from build123d import *

# Parameters (mm, degrees)
PROFILE_SKETCH_R              = 20.6375
PROFILE_EXTRUDE_DEPTH         = 3.175
BORE_SKETCH_R                 = 14.4145
BORE_CUT_DEPTH                = 4.175
BOLT_CLEARANCE_SKETCH_R       = 1.4732
BOLT_CLEARANCE_CUT_DEPTH      = 4.175
BOLT_HEAD_CLEARANCE_SKETCH_R  = 2.4511
BOLT_HEAD_CLEARANCE_CUT_DEPTH = 4.175


with BuildPart() as part:
    # Profile Sketch → Profile Extrude (new body)
    with BuildSketch(Plane(origin=(0, 0, 0), x_dir=(1, 0, 0), z_dir=(0, 1, 0))):
        Circle(PROFILE_SKETCH_R)
    extrude(amount=PROFILE_EXTRUDE_DEPTH)

    # Bore Sketch → Bore Cut (cut, through all)
    with BuildSketch(Plane(origin=(0, 0, 0), x_dir=(-1, 0, 0), z_dir=(0, -1, 0))):
        Circle(BORE_SKETCH_R)
    extrude(amount=-BORE_CUT_DEPTH, mode=Mode.SUBTRACT)

    # Bolt Clearance Sketch → Bolt Clearance Cut (cut, through all)
    with BuildSketch(Plane.XZ):
        with Locations((0, 17.526)):
            Circle(BOLT_CLEARANCE_SKETCH_R)
        with Locations((17.526, 0)):
            Circle(BOLT_CLEARANCE_SKETCH_R)
        with Locations((0, -17.526)):
            Circle(BOLT_CLEARANCE_SKETCH_R)
        with Locations((-17.526, 0)):
            Circle(BOLT_CLEARANCE_SKETCH_R)
    extrude(amount=-BOLT_CLEARANCE_CUT_DEPTH, mode=Mode.SUBTRACT)

    # Bolt Head Clearance Sketch → Bolt Head Clearance Cut (cut, through all)
    with BuildSketch(Plane(origin=(0, 0, 0), x_dir=(-1, 0, 0), z_dir=(0, -1, 0))):
        with Locations((-12.392753447, -12.392753447)):
            Circle(BOLT_HEAD_CLEARANCE_SKETCH_R)
        with Locations((-12.392753447, 12.392753447)):
            Circle(BOLT_HEAD_CLEARANCE_SKETCH_R)
        with Locations((12.392753447, 12.392753447)):
            Circle(BOLT_HEAD_CLEARANCE_SKETCH_R)
        with Locations((12.392753447, -12.392753447)):
            Circle(BOLT_HEAD_CLEARANCE_SKETCH_R)
    extrude(amount=-BOLT_HEAD_CLEARANCE_CUT_DEPTH, mode=Mode.SUBTRACT)


solid = part.part
Build history of the part. All positions in model axes, mm. Round coordinates to 2 decimals unless told otherwise and drop trailing zeros. Loops run counter-clockwise (first coordinate to the right, second up) from the corner with the lowest first, then second, coordinate; pieces in that order, holes last. Notation, with made-up numbers: (58, 29.5) -> (72, 29.5) arc R18 cw to (72, 45.5) -> close; hole circle Ø8 at (2.25, 0). An arc over 180 degrees is marked (long way). Answer in a Markdown table with one row per item.
Item 1: Drill centre lines: L1, parallel to Z at x = 0, y = 1.1; L2, parallel to Z at x = 10.5, y = 1.45; L3, parallel to X at y = 2.95, z = -0.5. Where is each one in solid material? Low to high. Write a range as [from, to].
Answers below:
| item | result |
|---|---|
| L1 | z = [-20.64, -19], [-16.05, -14.41], [14.41, 16.05], [19, 20.64] |
| L2 | z = [-17.77, -13.95], [-10.84, -9.88], [9.88, 10.84], [13.95, 17.77] |
| L3 | x = [-20.63, -18.91], [-16.14, -14.41], [14.41, 16.14], [18.91, 20.63] |
Item 2: Saw through at B-B (x = 0). Write the cut outline in (y, z) (1 decimal).
Answers below:
| item | result |
|---|---|
| outline | (0, -20.6) -> (3.2, -20.6) -> (3.2, -19) -> (0, -19) -> close; (0, -16.1) -> (3.2, -16.1) -> (3.2, -14.4) -> (0, -14.4) -> close; (0, 14.4) -> (3.2, 14.4) -> (3.2, 16.1) -> (0, 16.1) -> close; (0, 19) -> (3.2, 19) -> (3.2, 20.6) -> (0, 20.6) -> close |
Item 3: Saw through at C-C (y = 2.2). State how many separate pieces and enclosed holes the cut face has, and give its area (4 significant figures).
Answers below:
| item | result |
|---|---|
| separate pieces | 1 |
| enclosed holes | 9 |
| area | 582.5 mm² |
Item 4: Saw through at A-A (z = 0). Write the cut outline in (x, y) (1 decimal), and give its area (3 significant figures).
Answers below:
| item | result |
|---|---|
| outline | (-20.6, 0) -> (-19, 0) -> (-19, 3.2) -> (-20.6, 3.2) -> close; (-16.1, 0) -> (-14.4, 0) -> (-14.4, 3.2) -> (-16.1, 3.2) -> close; (14.4, 0) -> (16.1, 0) -> (16.1, 3.2) -> (14.4, 3.2) -> close; (19, 0) -> (20.6, 0) -> (20.6, 3.2) -> (19, 3.2) -> close |
| area | 20.8 mm² |
Item 5: Pin check, flat tips, straight feed: pin 1 (4.5 mm diameter, centred on x = 0, z = 17.526, fed in from +Y) (3 decimals); pin 2 (1 mm diameter, centred on x = -7.5, y = 1.5, fed in from +Z); pin 3 (1 mm diameter, centred on x = -8.5, y = 3, fed in from +Z). Stop position of each tip, or through.
Answers below:
| item | result |
|---|---|
| pin 1 | stops at y = 3.175 |
| pin 2 | stops at z = 19.41 |
| pin 3 | stops at z = 19.02 |
Item 6: Mould opens along Z. For faces 1 (the flat face through (-14, 0, -5)), 2 (the cylindrical face through (-1.47, 1.57, -17.46)), 3 (the cylindrical face through (-4.474, 1.565, 20.147)) say: +Z half, -Z half, draft (parallel to the pull), parting line (faces both ways), or undercut.
Answers below:
| item | result |
|---|---|
| face 1 | draft |
| face 2 | undercut |
| face 3 | parting line |
Item 7: Saw through at D-D (x = 9). Write the cut outline in (y, z) (3 decimals).
Answers below:
| item | result |
|---|---|
| outline | (0, -18.572) -> (3.175, -18.572) -> (3.175, -11.26) -> (0, -11.26) -> close; (0, 11.26) -> (3.175, 11.26) -> (3.175, 18.572) -> (0, 18.572) -> close |
